Can you work these out from the model? Positions are in its coordinate system, mm. Face numbers are marked on the shaded views. Coordinates: 2 decimals unless noted, no trailing zeros. Loops run counter-clockwise (first coordinate to the right, second up) from the corner with the lowest first, then second, coordinate; pieces in that order, holes last. Notation, with made-up numbers: M -11.75,5 L 33.25,5 A23 ccw 33.25,34 Z; hole C 79.5,59 d5. An arc over 180 degrees is marked long. Return JSON: item names as keys, results as strings. Group by question number.
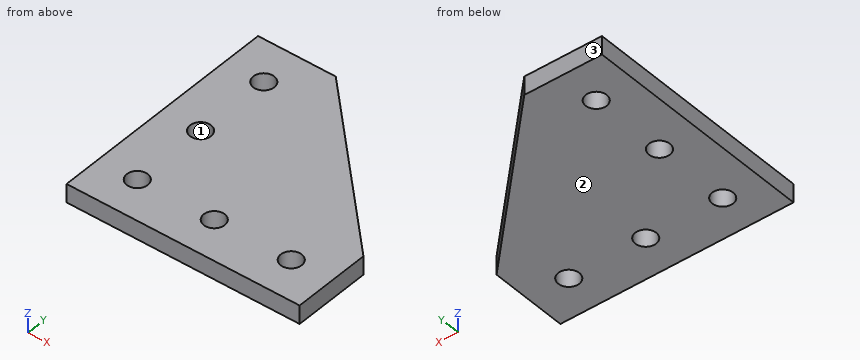
```python
from build123d import *

# Parameters (mm, degrees)
SKETCH1_R           = 2.7
BOSS_EXTRUDE1_DEPTH = 2.38125


with BuildPart() as part:
    # Sketch1 → Boss-Extrude1 (new, symmetric)
    with BuildSketch(Plane.XY):
        Polygon((0, 0), (0, 60), (20, 60), (60, 20), (60, 0), align=None)
        with Locations(Location((10, 10, 0), (0, 0, 180))):
            Circle(SKETCH1_R, mode=Mode.SUBTRACT)
        with Locations(Location((29.812, 10, 0), (0, 0, 180))):
            Circle(SKETCH1_R, mode=Mode.SUBTRACT)
        with Locations(Location((49.624, 10, 0), (0, 0, 180))):
            Circle(SKETCH1_R, mode=Mode.SUBTRACT)
        with Locations(Location((10, 29.812, 0), (0, 0, 180))):
            Circle(SKETCH1_R, mode=Mode.SUBTRACT)
        with Locations(Location((10, 49.624, 0), (0, 0, 180))):
            Circle(SKETCH1_R, mode=Mode.SUBTRACT)
    extrude(amount=BOSS_EXTRUDE1_DEPTH, both=True)


solid = part.part
```
1) Suppose I cut it at C-C, the plane z = 1.65. List the corners of the cut face in (x, y) for me.
2) Suppose I cut it at D-D, the plane y = 22. List the corners of the cut face in (x, z) for me, then the cut area to 3 significant figures.
3) If I drill on line 1 (Y direction, x = 10, z = -0.15); line 2 (X direction, y = 9.5, z = 0.9), over which ranges is the centre line in solid material (lowest first)? Write a range as from..to.
4) Suppose I cut it at A-A, the plane y = 10. List the corners of the cut face in (x, z) for me.
5) If we mould it in two halves opening along Y, with no side actions, what happens to the marked faces 1, 2 and 3? For each: +Y half, -Y half, draft (parallel to the pull), parting line (faces both ways), or undercut.
Returned:
{
 "1": {"outline": "M 0,0 L 60,0 L 60,20 L 20,60 L 0,60 Z; hole C 10,10 d5.4; hole C 10,29.81 d5.4; hole C 10,49.62 d5.4; hole C 29.81,10 d5.4; hole C 49.62,10 d5.4"},
 "2": {"outline": "M 0,-2.38 L 58,-2.38 L 58,2.38 L 0,2.38 Z", "area": "276 mm²"},
 "3": {"line 1": "y = 0..7.3, 12.7..27.11, 32.51..46.92, 52.32..60", "line 2": "x = 0..7.35, 12.65..27.16, 32.47..46.97, 52.28..60"},
 "4": {"outline": "M 0,-2.38 L 7.3,-2.38 L 7.3,2.38 L 0,2.38 Z; M 12.7,-2.38 L 27.11,-2.38 L 27.11,2.38 L 12.7,2.38 Z; M 32.51,-2.38 L 46.92,-2.38 L 46.92,2.38 L 32.51,2.38 Z; M 52.32,-2.38 L 60,-2.38 L 60,2.38 L 52.32,2.38 Z"},
 "5": {"face 1": "undercut", "face 2": "draft", "face 3": "+Y half"}
}
